Check sheet for the drawn part. Datum: minimum x, y, z corner. Units: mm. A direction names the side the tool comes from. Coordinates: 2 decimals unless noted, no trailing zeros. Loops run counter-clockwise (first coordinate to the right, second up) from the corner with the lowest first, then second, coordinate; pieces in that order, holes last.
Q1. Sectioned sample at D-D (z = 4.2). Enter the section's corners in (x, y), then the cut area to 3 significant figures.
Q2. Go/stop test with flat-tipped pins: P1, Ø1, axis at y = 4, z = 0.5, coming from the +X side; P2, Ø2, axis at x = 1, z = 2.5, coming from the +Y side. Record where each tip stops, or that it passes through.
Q3. Sectioned sample at A-A (y = 2.5). Enter the section's corners in (x, z).
Q4. Access from +Z, -Z, +X, -X, +Y, -Y to the whole of each face (thin tool, end or side, straight path). Record for the marked faces 4 and 5.
Q5. Sectioned sample at C-C (z = 3.7). Enter the section's corners in (x, y).
Q6. Mould release check, pull along X, two halves, no side actions. Record for the marked faces 1, 2 and 3: +X half, -X half, draft (parallel to the pull), parting line (faces both ways), or undercut.
Q7. Material ranges on probe 1 along Y at (x, z) = (2.5, 1.8); probe 2 along Z at (x, y) = (1.75, 2.1); probe 3 along X at (y, z) = (3, 2.05), recorded low to high.
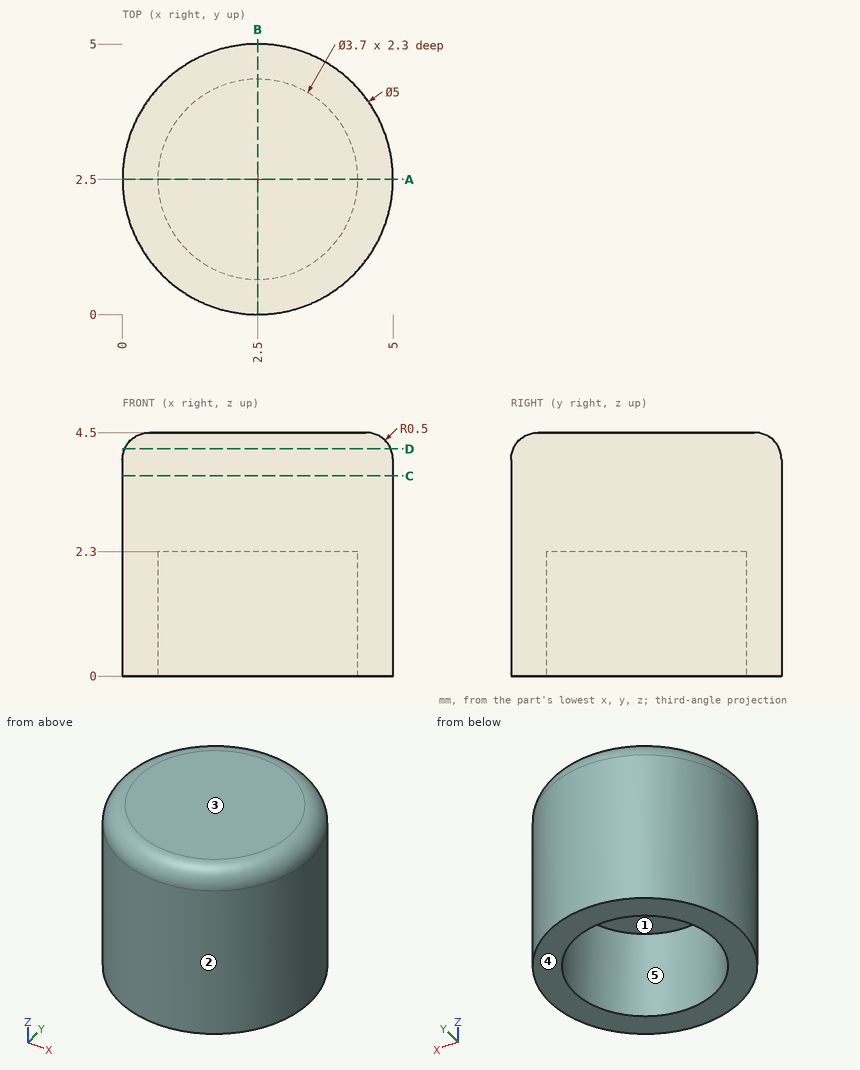
Geometry check:
1. outline: circle Ø4.92 at (2.5, 2.5)
1. area: 19.0 mm2
2. P1: stops at x = 4.79
2. P2: stops at y = 4.95
3. outline: (0, 0) - (0.65, 0) - (0.65, 2.3) - (4.35, 2.3) - (4.35, 0) - (5, 0) - (5, 4) arc R0.5 ccw to (4.5, 4.5) - (0.5, 4.5) arc R0.5 ccw to (0, 4) - close
4. face 4: -Z, +X, -X, +Y, -Y
4. face 5: -Z
5. outline: circle Ø5 at (2.5, 2.5)
6. face 1: undercut
6. face 2: parting line
6. face 3: draft
7. probe 1: y = 0 to 0.65, 4.35 to 5
7. probe 2: z = 2.3 to 4.5
7. probe 3: x = 0.05 to 0.72, 4.28 to 4.95
